For this review, use the dimensioned drawing (mm, ordinates from the lowest corner) and the shaded views. Give positions to 0.01 mm unless a question says otherwise; leave off trailing zeros. Order: outer loops, then holes, each group sorted by start corner. A loop starts at its lowest first (then second) coordinate and runs counter-clockwise, first axis right, second up. Notation, with made-up numbers: (80.5, -12.75) - (99.5, -12.75) arc R28 ccw to (99.5, 12.25) - close; hole circle Ø7 at (-37, 10.5). An arc over 180 degrees is marked (long way). One line per item, written item: value.
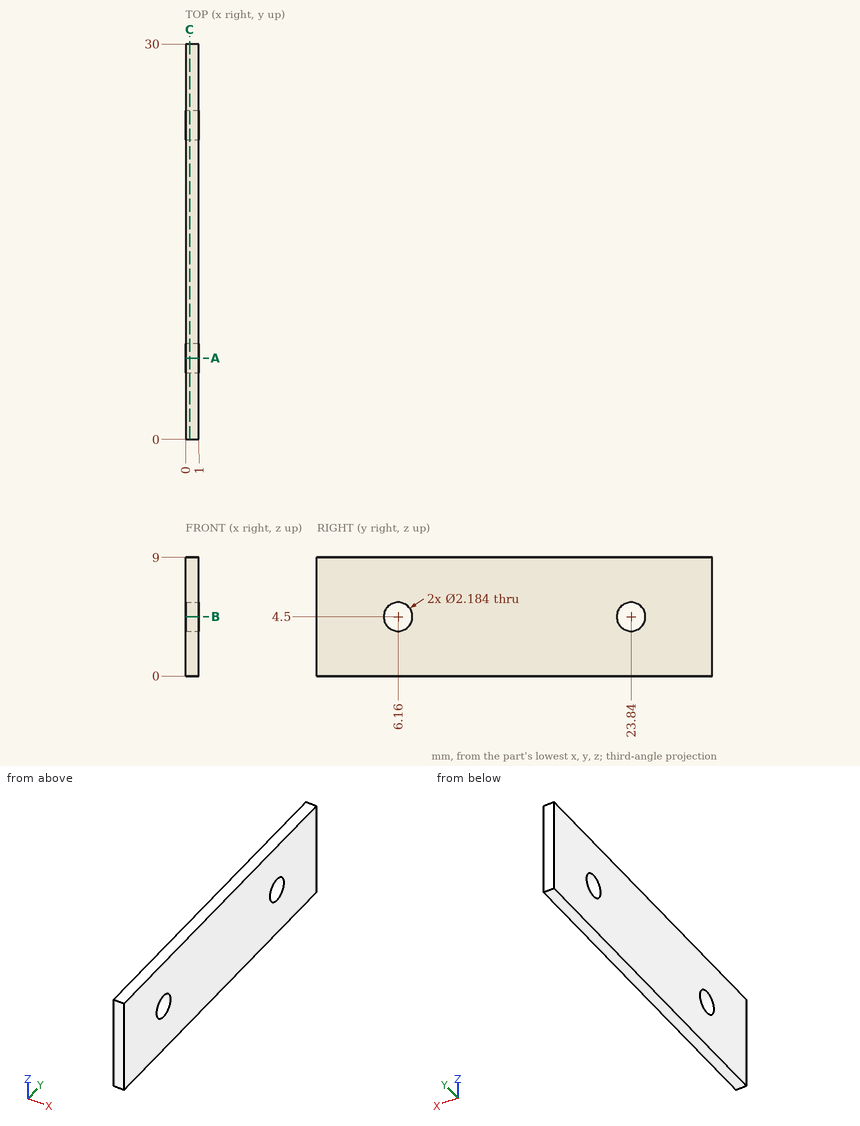
(1) For P1, Ø1.7, axis at y = 6.16, z = 4.5, coming from the -X side, flat-tipped, find the tip position at first contact; note if it passes through.
Answers below:
P1: passes through
(2) Take a section at B-B (z = 4.5). Write out the cut boundary in (x, y).
Answers below:
outline: (0, 0) - (1, 0) - (1, 5.07) - (0, 5.07) - close; (0, 7.25) - (1, 7.25) - (1, 22.75) - (0, 22.75) - close; (0, 24.93) - (1, 24.93) - (1, 30) - (0, 30) - close
(3) Take a section at A-A (y = 6.16). Write out the cut boundary in (x, z).
Answers below:
outline: (0, 0) - (1, 0) - (1, 3.41) - (0, 3.41) - close; (0, 5.59) - (1, 5.59) - (1, 9) - (0, 9) - close
(4) Take a section at C-C (x = 0.3). Write out the cut boundary in (y, z) (1 decimal).
Answers below:
outline: (0, 0) - (30, 0) - (30, 9) - (0, 9) - close; hole circle Ø2.2 at (6.2, 4.5); hole circle Ø2.2 at (23.8, 4.5)
(5) Wall thickness on line 1 (Z direction, x = 0.8, y = 6.16); line 2 (Y direction, x = 0.3, z = 5); line 3 (Y direction, x = 0.05, z = 4.25): over which ranges is each line inside the solid? List them lowest first. Write a range as from..to.
Answers below:
line 1: z = 0..3.41, 5.59..9
line 2: y = 0..5.19, 7.13..22.87, 24.81..30
line 3: y = 0..5.1, 7.22..22.78, 24.9..30
